The model under review builds one solid part; all positions refer to its coordinate system, in mm. A direction names the side the tool comes from. Round coordinates to 2 decimals unless told otherwise and drop trailing zeros. Loops run counter-clockwise (first coordinate to the right, second up) from the corner with the lowest first, then second, coordinate; pieces in that order, holes last. Notation, with made-up numbers: M 28,40 L 48,40 A27 cw 48,76 Z; hole C 55,86 d10. An arc over 180 degrees is marked long. One line per question, with ' | ' between items.
from build123d import *

# Parameters (mm, degrees)
SKETCH1_W            = 55
SKETCH1_H            = 70.86
SKETCH1_W_2          = 39
SKETCH1_H_2          = 19
BOSS_EXTRUDE1_DEPTH  = 6.35
SKETCH12_R           = 7.94
BOSS_EXTRUDE11_DEPTH = 6.35
BOSS_EXTRUDE14_START = -6.35
BOSS_EXTRUDE14_DEPTH = 6.35
SKETCH15_W           = 23
SKETCH15_H           = 70.86
BOSS_EXTRUDE13_DEPTH = 6.35
FILLET2_R            = 16.38
FILLET3_R            = 6.35
CUT_EXTRUDE1_REACH   = 92.618
SKETCH17_R           = 4.625


with BuildPart() as part:
    # Sketch1 → Boss-Extrude1 (new body)
    with BuildSketch(Plane(origin=(0, 0, 0), x_dir=(1, 0, 0), z_dir=(0, 1, 0))):
        with Locations((0, 15)):
            Rectangle(SKETCH1_W, SKETCH1_H)
        Rectangle(SKETCH1_W_2, SKETCH1_H_2, mode=Mode.SUBTRACT)
    extrude(amount=BOSS_EXTRUDE1_DEPTH)

    # Sketch12 → Boss-Extrude11 (add)
    with BuildSketch(Plane.XY.offset(-50.43)):
        with BuildLine():
            Line((16, 22.728660684), (16, 6.35))
            Line((16, 6.35), (-16, 6.35))
            Line((-16, 6.35), (-16, 22.728660684))
            ThreePointArc((-16, 22.728660684), (0, 38.728660684), (16, 22.728660684))
        make_face()
        with Locations((0, 22.728660684)):
            Circle(SKETCH12_R, mode=Mode.SUBTRACT)
    extrude(amount=BOSS_EXTRUDE11_DEPTH)

    # Sketch16 → Boss-Extrude14 (add)
    with BuildSketch(Plane.XY.offset(20.43).offset(BOSS_EXTRUDE14_START)):
        with BuildLine():
            Line((-16, 6.35), (-16, 22.728660684))
            ThreePointArc((-16, 22.728660684), (0, 38.728660684), (16, 22.728660684))
            Line((16, 22.728660684), (16, 6.35))
            Line((16, 6.35), (-16, 6.35))
        make_face()
    extrude(amount=BOSS_EXTRUDE14_DEPTH)

    # Sketch15 → Boss-Extrude13 (add)
    with BuildSketch(Plane(origin=(0, 6.35, 0), x_dir=(1, 0, 0), z_dir=(0, 1, 0))):
        with Locations((-39, 15)):
            Rectangle(SKETCH15_W, SKETCH15_H)
    extrude(amount=-BOSS_EXTRUDE13_DEPTH)

    # Fillet2
    # the kernel refuses this fillet: 16.38 mm, written as the material it adds along each edge
    with BuildSketch(Plane(origin=(16, 6.35, -50.43), x_dir=(0, 1, 0), z_dir=(0, 0, 1)), Plane(origin=(16, 6.35, 14.08), x_dir=(0, 1, 0), z_dir=(0, 0, 1))) as fillet2_piece_1:
        with BuildLine():
            CenterArc((15.636176003, -16.38), FILLET2_R, 90, 72.667025782)
            Line((0, -11.5), (0, 0))
            Line((0, 0), (15.636176003, 0))
        make_face()
    fillet2_piece_1_solid = extrude(amount=6.35, mode=Mode.PRIVATE)
    with BuildSketch(Plane(origin=(-16, 6.35, 14.08), x_dir=(8.356150350670102e-10, 1.0, 0), z_dir=(0, 0, 1)), Plane(origin=(-16, 6.35, -50.43), x_dir=(8.356150350670102e-10, 1.0, 0), z_dir=(0, 0, 1))) as fillet2_piece_2:
        with BuildLine():
            CenterArc((16.379999986, 16.379999986), FILLET2_R, 180.000000048, 89.997630107)
            Line((-1.4e-08, 16.379999972), (-1.638000014, 16.379999971))
            Line((-1.638000014, 16.379999971), (-1.637999999, -1.638000001))
            Line((-1.637999999, -1.638000001), (16.379254733, -1.637999999))
            Line((16.379254733, -1.637999999), (16.379322483, 0))
        make_face()
    fillet2_piece_2_solid = extrude(amount=6.35, mode=Mode.PRIVATE)
    add([fillet2_piece_1_solid, fillet2_piece_2_solid])

    # Fillet3
    fillet3_edges = [part.edges().sort_by_distance(p)[0] for p in [
        (27.5, 3.175, -50.43),
        (27.5, 3.175, 20.43),
        (-50.5, 3.175, 20.43),
        (-50.5, 3.175, -50.43),
    ]]
    fillet(fillet3_edges, radius=FILLET3_R)

    # Sketch17 → Cut-Extrude1 (cut, up to next)
    with BuildSketch(Plane(origin=(0, 0, 14.08), x_dir=(-1, 0, 0), z_dir=(0, 0, -1)), mode=Mode.PRIVATE) as cut_extrude1_sk1:
        with Locations((0, 22.728660684)):
            Circle(SKETCH17_R)
    cut_extrude1_tool1 = extrude(cut_extrude1_sk1.sketch, amount=-CUT_EXTRUDE1_REACH, mode=Mode.PRIVATE) & part.part
    add(cut_extrude1_tool1.solids().sort_by_distance((0, 22.728661, 14.08))[0], mode=Mode.SUBTRACT)


solid = part.part
1) Insertion check: P1, Ø3, axis at x = -13.5, z = -10.5, coming from the +Y side. The pin has a flat end and moves straight along its axis. Give the tip position at first contact, or say it passes through.
Output values:
P1: stops at y = 6.35
2) Add section B-B on y = 28.5. State the section outline as (x, z) points, then the cut area to 3 significant figures.
Output values:
outline: M -14.92,-50.43 L -5.45,-50.43 L -5.45,-44.08 L -14.92,-44.08 Z; M -14.92,14.08 L 14.92,14.08 L 14.92,20.43 L -14.92,20.43 Z; M 5.45,-50.43 L 14.92,-50.43 L 14.92,-44.08 L 5.45,-44.08 Z | area: 310 mm²
3) Add section D-D on y = 4.5. State the section outline as (x, z) points, then the cut area to 3 significant figures.
Output values:
outline: M -50.5,-44.08 A6.35 ccw -44.15,-50.43 L 21.15,-50.43 A6.35 ccw 27.5,-44.08 L 27.5,14.08 A6.35 ccw 21.15,20.43 L -44.15,20.43 A6.35 ccw -50.5,14.08 Z; hole M -19.5,-9.5 L 19.5,-9.5 L 19.5,9.5 L -19.5,9.5 Z | area: 4,750 mm²
4) For line 1 (Y direction, x = 0, z = -46); line 2 (Z direction, x = 16, y = 10.5); line 3 (Z direction, x = -15, y = 2.5), list the stretches that pass through material, from the lowest coordinate up.
Output values:
line 1: y = 0 to 14.79, 30.67 to 38.73 | line 2: z = -50.43 to -44.08, 14.08 to 20.43 | line 3: z = -50.43 to -9.5, 9.5 to 20.43
5) Machinability: for faces 5 (the flat face through (19.5, 3, 0)), 6 (the cylindrical face through (25.59, 3.98, 18.62)), 7 (the cylindrical face through (3.664, 15.685, -47.299)), which of the approach directions +Z, -Z, +X, -X, +Y, -Y give a long, thin tool a straight path to every point of the face, cutting with its end or side? Answer none if there is none.
Output values:
face 5: +Y, -Y | face 6: +Z, +X, +Y, -Y | face 7: -Z
6) Add section A-A on x = 0. State the section outline as (y, z) points, then the cut area to 3 significant figures.
Output values:
outline: M 0,-50.43 L 14.79,-50.43 L 14.79,-44.08 L 6.35,-44.08 L 6.35,-9.5 L 0,-9.5 Z; M 0,9.5 L 6.35,9.5 L 6.35,14.08 L 18.1,14.08 L 18.1,20.43 L 0,20.43 Z; M 27.35,14.08 L 38.73,14.08 L 38.73,20.43 L 27.35,20.43 Z; M 30.67,-50.43 L 38.73,-50.43 L 38.73,-44.08 L 30.67,-44.08 Z | area: 581 mm²
7) Mouldability with a two-part tool opening along Z and no side actions: class faces 1 (the flat face through (-19.5, 3, 0)), 2 (the flat face through (-5, 15, -50.43)), 3 (the cylindrical face through (-20.926, 11.02, 17.211)), 4 (the cylindrical face through (-48.59, 3.13, 18.62)) as +Z half, -Z half, draft (parallel to the pull), parting line (faces both ways), or undercut.
Output values:
face 1: undercut | face 2: -Z half | face 3: draft | face 4: +Z half
8) Add section C-C on x = -17.5. State the section outline as (y, z) points, then the cut area to 3 significant figures.
Output values:
outline: M 0,-50.43 L 15.88,-50.43 L 15.88,-44.08 L 6.35,-44.08 L 6.35,-9.5 L 0,-9.5 Z; M 0,9.5 L 6.35,9.5 L 6.35,14.08 L 15.88,14.08 L 15.88,20.43 L 0,20.43 Z | area: 450 mm²
